The listing builds one solid part. Answer for the finished solid, in the listing's coordinates (mm). Face numbers are marked on the shaded views. A direction names the side the tool comes from. Round coordinates to 2 decimals unless told otherwise and drop trailing zeros. Write each loop counter-clockwise with the first axis right and the second up, starting at its lowest first coordinate (ties: lowest second). Pieces come first, ordered by that corner, then holes. Notation, with made-up numbers: M 26,6 L 57,6 A14 ccw 57,18 Z; hole C -6.75,85 d4. An arc over 180 degrees is marked long. Write each question's results on one line, items separated by ' | '.
from build123d import *

# Parameters (mm, degrees)
F1_DEPTH       = 4
F2_D           = 3.2
F2_CBORE_D     = 6
F2_CBORE_DEPTH = 2
F3_D           = 5.2
F4_R           = 3


with BuildPart() as f1:
    # F0 (on Front) → F1 (new body)
    with BuildSketch(Plane.XZ):
        Polygon((0, -9), (-16, -9), (-16, -41), (0, -41), (0, -44), (0, -50), (9, -50), (9, 0), (0, 0), (0, -6), align=None)
    extrude(amount=F1_DEPTH)

    # F2 (through all)
    with Locations(Plane(origin=(0, 0, 0), x_dir=(1, 0, 0), z_dir=(0, 1, 0))):
        with Locations((4.5, 4.5), (4.5, 45.5)):
            CounterBoreHole(F2_D / 2, F2_CBORE_D / 2, F2_CBORE_DEPTH)

    # F3 (through all)
    with Locations(Plane(origin=(0, 0, 0), x_dir=(1, 0, 0), z_dir=(0, 1, 0))):
        with Locations((-10, 15), (-10, 35)):
            Hole(F3_D / 2)

    # F4
    f4_edges = [f1.edges().sort_by_distance(p)[0] for p in [
        (-16, -2, -9),
        (-16, -2, -41),
        (9, -2, 0),
        (0, -2, 0),
        (0, -2, -50),
        (9, -2, -50),
    ]]
    fillet(f4_edges, radius=F4_R)


solid = f1.part
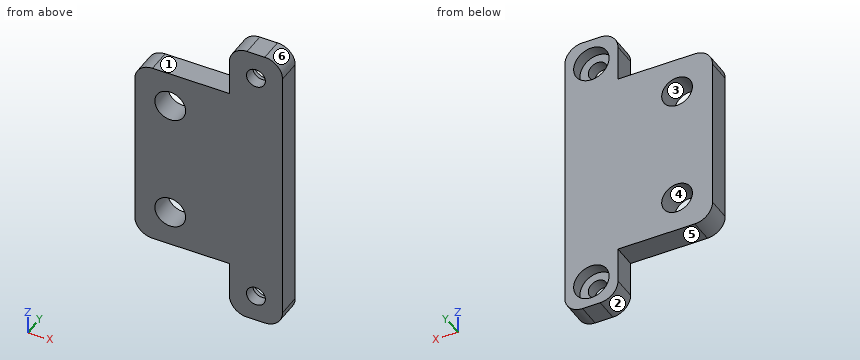
1) The mould has two halves that part along X. Classify the marked faces 3, 4, 5 and 6: +X half, -X half, draft (parallel to the pull), parting line (faces both ways), or undercut.
Return value:
face 3: undercut | face 4: undercut | face 5: draft | face 6: +X half
2) Section B-B (x = -10) is taken. Determine the outline of the cut face in (y, z), then the cut area to 3 significant figures.
Return value:
outline: M -4,-41 L 0,-41 L 0,-37.6 L -4,-37.6 Z; M -4,-32.4 L 0,-32.4 L 0,-17.6 L -4,-17.6 Z; M -4,-12.4 L 0,-12.4 L 0,-9 L -4,-9 Z | area: 86.4 mm²
3) Section A-A (z = -15) is taken. Determine the outline of the cut face in (x, y), then the cut area to 3 significant figures.
Return value:
outline: M -16,-4 L -12.6,-4 L -12.6,0 L -16,0 Z; M -7.4,-4 L 9,-4 L 9,0 L -7.4,0 Z | area: 79.2 mm²
4) A tool of negligible diameter and unlimited length cuts with its end or side. For the marked faces 1 and 2, from which of +Z, -Z, +X, -X, +Y, -Y can it reach the whole face along a straight path? Write none if from no direction.
Return value:
face 1: +Z, -X, +Y, -Y | face 2: -Z, -X, +Y, -Y
5) Section C-C (y = -0.8) is taken. Determine the outline of the cut face in (x, z), then the cut area to 3 significant figures.
Return value:
outline: M -16,-38 A3 ccw -13,-41 L 0,-41 L 0,-47 A3 ccw 3,-50 L 6,-50 A3 ccw 9,-47 L 9,-3 A3 ccw 6,0 L 3,0 A3 ccw 0,-3 L 0,-9 L -13,-9 A3 ccw -16,-12 Z; hole C -10,-35 d5.2; hole C -10,-15 d5.2; hole C 4.5,-45.5 d6; hole C 4.5,-4.5 d6 | area: 851 mm²
6) Find the intervals of material crossed by line 1 (Z direction, x = 4.5, y = -0.55); line 2 (Z direction, x = -10, y = -0.9); line 3 (X direction, y = -3.1, z = -8), in increasing order.
Return value:
line 1: -50 to -48.5, -42.5 to -7.5, -1.5 to 0 | line 2: -41 to -37.6, -32.4 to -17.6, -12.4 to -9 | line 3: 0 to 9
7) Each of these flat-tipped pins is pushed along its axis until it touches: pin 1 (1 mm diameter, centred on x = -2, y = -2, fed in from -Z); pin 2 (2 mm diameter, centred on x = -5, y = -1.5, fed in from +Z); pin 3 (1.2 mm diameter, centred on y = -1.5, z = -5, fed in from -X). Where does it stop, or does it pass through?
Return value:
pin 1: z = -41 | pin 2: z = -9 | pin 3: x = 0
8) Section D-D (z = -34) is taken. Determine the outline of the cut face in (x, y), then the cut area to 3 significant figures.
Return value:
outline: M -16,-4 L -12.4,-4 L -12.4,0 L -16,0 Z; M -7.6,-4 L 9,-4 L 9,0 L -7.6,0 Z | area: 80.8 mm²
